Source: CAD feature listing. Evaluate the final solid. Frame: model axes, mm. A direction names the side the tool comes from. Round coordinates to 2 decimals unless told otherwise and drop trailing zeros. Write each loop counter-clockwise with the first axis right and the second up, starting at its lowest first coordinate (ties: lowest second). Pieces come first, ordered by that corner, then holes. Notation, with made-up numbers: (-3, 79.5) - (53, 79.5) arc R31 cw to (53, 117.5) - close; hole circle Ø4 at (25, 21). An arc over 180 degrees is marked (long way). Write item = value, one per line. Start each with the question number.
```python
from build123d import *

# Parameters (mm, degrees)
F0_R      = 284.48
F0_R_2    = 107.1929715192
F0_R_3    = 113.5568544934
F1_DEPTH  = 43.18
F2_DEPTH  = 25.4
F3_R      = 188.583728209
F4_DEPTH  = 83.82
F5_R      = 191.3062955449
F6_DEPTH  = 25.4
F7_DEPTH  = 50.8
F8_R      = 44.4860383671
F8_R_2    = 42.5130720405
F9_DEPTH  = 73.66
F11_R     = 25.0558665745
F12_DEPTH = 96.52
F13_R     = 24.5435955791
F15_DEPTH = 60.96
F16_R     = 25.0526065755
F17_DEPTH = 25.4
F18_R     = 25.0571
F18_R_2   = 24.5435955791
F19_DEPTH = 25.4


# Not quite as in the source:
# - the program builds the solid bodies; features that only make, move or delete a surface that nothing else refers to are left out


with BuildPart() as f1:
    # F0 (on Top) → F1 (new body)
    with BuildSketch(Plane.XY):
        Circle(F0_R)
        with Locations((-137.995660305, 0)):
            Circle(F0_R_2, mode=Mode.SUBTRACT)
        with Locations((127.078294754, 0)):
            Circle(F0_R_3, mode=Mode.SUBTRACT)
        with BuildLine():
            ThreePointArc((-102.7708947659, 136.166498065), (-10.3978756011, 204.9943768322), (94.8023349047, 158.0585986376))
            ThreePointArc((94.8023349047, 158.0585986376), (-4.0832297138, 148.0055566847), (-102.7708947659, 136.166498065))
        make_face(mode=Mode.SUBTRACT)
        with Locations((-137.995660305, 0)):
            Circle(F0_R_2)
        with Locations((127.078294754, 0)):
            Circle(F0_R_3)
        with BuildLine():
            ThreePointArc((-102.7708947659, 136.166498065), (-4.0832297138, 148.0055566847), (94.8023349047, 158.0585986376))
            ThreePointArc((94.8023349047, 158.0585986376), (-10.3978756011, 204.9943768322), (-102.7708947659, 136.166498065))
        make_face()
    extrude(amount=F1_DEPTH)

    # F2 (add): a face of the model
    f2_faces = [f1.faces().sort_by_distance(p)[0] for p in [
        (0, 0, 0),
    ]]
    extrude(f2_faces, amount=F2_DEPTH)

    # F3 (on face) → F4 (join)
    with BuildSketch(Plane(origin=(0, 0, -25.4), x_dir=(1, 0, 0), z_dir=(0, 0, -1))):
        with Locations((12.9366638139, 0)):
            Circle(F3_R)
    extrude(amount=-F4_DEPTH)

    # F5 (on face) → F6 (join)
    with BuildSketch(Plane(origin=(0, 0, -25.4), x_dir=(1, 0, 0), z_dir=(0, 0, -1))):
        with Locations((18.2807631791, 0)):
            Circle(F5_R)
    extrude(amount=F6_DEPTH)

    # F7 (add): faces of the model
    f7_faces = [f1.faces().sort_by_distance(p)[0] for p in [
        (-276.4336905155, 0, -25.4),
        (-173.3657778507, 0, -25.4),
        (18.2807631791, 0, -50.8),
    ]]
    extrude(f7_faces, amount=F7_DEPTH)

    # F8 (on face) → F9 (join)
    with BuildSketch(Plane(origin=(0, 0, -101.6), x_dir=(1, 0, 0), z_dir=(0, 0, -1))):
        with Locations((-52.0154200494, 69.075293839)):
            Circle(F8_R)
        with Locations((109.2234924436, 57.04626441)):
            Circle(F8_R_2)
    extrude(amount=F9_DEPTH)

    # F11 (on face) → F12 (join)
    with BuildSketch(Plane(origin=(0, 0, -175.26), x_dir=(1, 0, 0), z_dir=(0, 0, -1))):
        with Locations((-52.0154200494, 69.075293839)):
            Circle(F11_R)
    extrude(amount=-F12_DEPTH)

    # F13 (on face) → F15 (join)
    with BuildSketch(Plane(origin=(0, 0, -175.26), x_dir=(1, 0, 0), z_dir=(0, 0, -1))):
        with Locations((-52.0154200494, 69.075293839)):
            Circle(F13_R)
    extrude(amount=-F15_DEPTH)

    # F16 (on face) → F17 (join)
    with BuildSketch(Plane(origin=(0, 0, -175.26), x_dir=(1, 0, 0), z_dir=(0, 0, -1))):
        with Locations((109.2234924436, 57.04626441)):
            Circle(F16_R)
    extrude(amount=F17_DEPTH)

    # F18 (on face) → F19 (join)
    with BuildSketch(Plane(origin=(0, 0, -175.26), x_dir=(1, 0, 0), z_dir=(0, 0, -1))):
        with Locations((-52.0154200494, 69.075293839)):
            Circle(F18_R)
        with Locations((-52.0154200494, 69.075293839)):
            Circle(F18_R_2, mode=Mode.SUBTRACT)
        with Locations((-52.0154200494, 69.075293839)):
            Circle(F18_R_2)
    extrude(amount=F19_DEPTH)


solid = f1.part
```
(1) Ray query, L1, parallel to Z at x = 3.5, y = -206; L2, parallel to X at y = -55.5, z = -113; L3, parallel to X at y = -73, z = -170. Return the intervals inside material, ascending. Write a range as from..to.
(2) Section C-C (x = 143). Return the cut outline in (y, z), plus the area to 3 significant figures.
(3) Section D-D (x = 0). Return the cut outline in (y, z).
(4) Contact query for flat-ended pins moving along their axis: P1, Ø3, axis at x = 63, y = 192.5, coming from the +Z side; P2, Ø1, axis at y = -32.5, z = -127.5, coming from the -X side; P3, Ø10, axis at x = 191.5, y = 215.5, coming from the -Z side. Output: stop coordinate, or through.
(5) Reachability of faces 4 (the flat face through (109, -57, -200.66)), 5 (the cylindrical face through (-28.1, -106.586, -137.914)), 6 (the flat face through (-130, 130, 43.18)) from +Z, -Z, +X, -X, +Y, -Y: full face, straight path, thin tool, end or side. Return the list, or none.
(6) Section B-B (z = -33). Return the cut outline in (x, y).
(7) Section A-A (y = 49). Return the cut outline in (x, z).
(8) Pull-direction query (X, two-part tool) for faces 1 (the cylindrical face through (-11.61, -186.98, 50.69)), 2 (the flat face through (-130, 122, -76.2)), 3 (the flat face through (-33, -50, -175.26)); classes: +X half, -X half, draft (parallel to the pull), parting line (faces both ways), or undercut.
Solution:
q1.L1 = -76.2..43.18
q1.L2 = -94.38..-9.65, 66.74..151.71
q1.L3 = -96.33..-7.7, 69.82..148.63
q2.outline = (-245.93, -76.2) - (-145.06, -76.2) - (-145.06, -101.6) - (-82.86, -101.6) - (-82.86, -175.26) - (-31.23, -175.26) - (-31.23, -101.6) - (145.06, -101.6) - (145.06, -76.2) - (245.93, -76.2) - (245.93, 43.18) - (136.56, 43.18) - (136.56, 58.42) - (-136.56, 58.42) - (-136.56, 43.18) - (-245.93, 43.18) - close
q2.area = 74,100 mm^2
q3.outline = (-284.48, -76.2) - (-190.43, -76.2) - (-190.43, -101.6) - (190.43, -101.6) - (190.43, -76.2) - (284.48, -76.2) - (284.48, 43.18) - (188.14, 43.18) - (188.14, 58.42) - (-188.14, 58.42) - (-188.14, 43.18) - (-284.48, 43.18) - close
q4.P1 = 43.18
q4.P2 = -78.05
q4.P3 = -76.2
q5.face_4 = -Z, +X, -X, +Y, -Y
q5.face_5 = -Z
q5.face_6 = +Z
q6.outline = circle Ø568.96 at (0, 0)
q7.outline = (-280.23, -76.2) - (-166.64, -76.2) - (-166.64, -101.6) - (203.21, -101.6) - (203.21, -76.2) - (280.23, -76.2) - (280.23, 43.18) - (195.04, 43.18) - (195.04, 58.42) - (-169.17, 58.42) - (-169.17, 43.18) - (-280.23, 43.18) - close
q8.face_1 = parting line
q8.face_2 = draft
q8.face_3 = undercut
